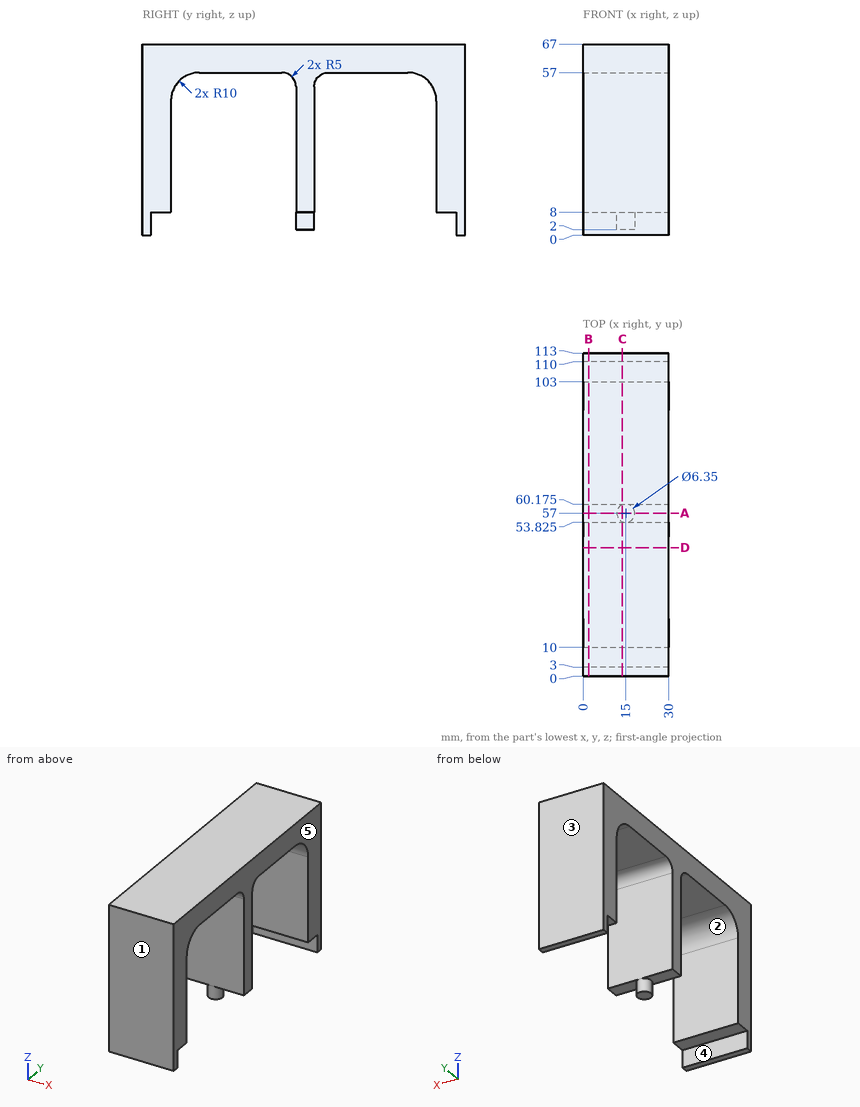
Design review of the part shown in the three views and the two pictorial views. Dimensions are in mm from the part's minimum x, y and z. A direction names the side the tool comes from. Round coordinates to 2 decimals unless told otherwise and drop trailing zeros. Loops run counter-clockwise (first coordinate to the right, second up) from the corner with the lowest first, then second, coordinate; pieces in that order, holes last.
(1) We need section B-B (x = 2). Give the boundary of the cut face in (y, z) (3 decimals).
Returned:
outline: (0, 0) - (3, 0) - (3, 8) - (10, 8) - (10, 47) arc R10 cw to (20, 57) - (48.825, 57) arc R5 cw to (53.825, 52) - (53.825, 8) - (60.175, 8) - (60.175, 52) arc R5 cw to (65.175, 57) - (93, 57) arc R10 cw to (103, 47) - (103, 8) - (110, 8) - (110, 0) - (113, 0) - (113, 67) - (0, 67) - close
(2) Clearance check with flat-ended pins moving along their axes: P1, Ø2, axis at x = 26.5, z = 55.5, coming from the -Y side; P2, Ø1.9, axis at x = 4.5, y = 57.5, coming from the -Z side; P3, Ø7, axis at x = 15, y = 58, coming from the -Z side; P4, Ø10, axis at x = 13.5, y = 37, coming from the -Z side. State where each tip first meets the part, or that it passes through.
Returned:
P1: stops at y = 0
P2: stops at z = 8
P3: stops at z = 2
P4: stops at z = 57
(3) Tool access review of the marked faces 1 and 2: name each direction out of +Z, -Z, +X, -X, +Y, -Y from which nothing blocks a thin tool from reaching the whole face with its end or side.
Returned:
face 1: +Z, -Z, +X, -X, -Y
face 2: -Z, +X, -X
(4) Mouldability with a two-part tool opening along Y and no side actions: class the marked faces 3, 4 and 5 as released by +Y, released by -Y, zero draft, split by the parting line, or undercut.
Returned:
face 3: released by +Y
face 4: undercut
face 5: zero draft
(5) We need section D-D (y = 45). Give the boundary of the cut face in (x, z).
Returned:
outline: (0, 57) - (30, 57) - (30, 67) - (0, 67) - close
(6) Wall thickness on line 1 along Y through (x, z) = (19.75, 43) (3 decimals); line 2 along Y through (x, z) = (9.5, 55.5); line 3 along Y through (x, z) = (3.75, 4.5): over which ranges is each line inside the solid? List them lowest first.
Returned:
line 1: y = 0 to 10, 53.825 to 60.175, 103 to 113
line 2: y = 0 to 14.73, 52.4 to 61.6, 98.27 to 113
line 3: y = 0 to 3, 110 to 113
(7) We need section C-C (x = 13.75). Give the boundary of the cut face in (y, z) (3 decimals).
Returned:
outline: (0, 0) - (3, 0) - (3, 8) - (10, 8) - (10, 47) arc R10 cw to (20, 57) - (48.825, 57) arc R5 cw to (53.825, 52) - (53.825, 8) - (54.081, 8) - (54.081, 2) - (59.919, 2) - (59.919, 8) - (60.175, 8) - (60.175, 52) arc R5 cw to (65.175, 57) - (93, 57) arc R10 cw to (103, 47) - (103, 8) - (110, 8) - (110, 0) - (113, 0) - (113, 67) - (0, 67) - close
(8) We need section A-A (y = 57). Give the boundary of the cut face in (x, z) (3 decimals), plus the area to 3 significant figures.
Returned:
outline: (0, 8) - (11.825, 8) - (11.825, 2) - (18.175, 2) - (18.175, 8) - (30, 8) - (30, 67) - (0, 67) - close
area: 1,810 mm2
